from build123d import *

# Parameters (mm, degrees)
SKETCH1_W           = 498.348
SKETCH1_H           = 165.1
BOSS_EXTRUDE1_DEPTH = 1.5875
BOSS_EXTRUDE2_DEPTH = 3.175
CUT_EXTRUDE1_DEPTH  = 286.681383539
LPATTERN1_COUNT     = 5
LPATTERN1_PITCH     = 88.9
CUT_EXTRUDE2_DEPTH  = 286.681383539
LPATTERN2_COUNT     = 2
LPATTERN2_PITCH     = 38.1


with BuildPart() as part:
    # Sketch1 → Boss-Extrude1 (new, symmetric)
    with BuildSketch(Plane(origin=(0, 0, 0), x_dir=(0, 0, -1), z_dir=(1, 0, 0))):
        Rectangle(SKETCH1_W, SKETCH1_H)
    extrude(amount=BOSS_EXTRUDE1_DEPTH, both=True)

    # Sketch2 → Boss-Extrude2 (add)
    with BuildSketch(Plane(origin=(1.5875, 0, 0), x_dir=(0, 0, -1), z_dir=(1, 0, 0))):
        Polygon((192.024, -139.7), (249.174, -82.55), (-249.174, -82.55), (-249.174, -139.7), align=None)
    extrude(amount=-BOSS_EXTRUDE2_DEPTH)

    # Sketch3 → Cut-Extrude1 (cut, through all)
    with BuildSketch(Plane.ZY.offset(1.5875)):
        with BuildLine():
            ThreePointArc((222.877, -130.81), (216.603382579, -128.211382579), (219.202, -134.485))
            Line((219.202, -134.485), (219.202, -130.81))
            Line((219.202, -130.81), (222.877, -130.81))
        make_face()
        with BuildLine():
            Line((219.202, -130.81), (219.202, -134.485))
            ThreePointArc((219.202, -134.485), (221.800617421, -133.408617421), (222.877, -130.81))
            Line((222.877, -130.81), (219.202, -130.81))
        make_face()
    cut_extrude1 = extrude(amount=-CUT_EXTRUDE1_DEPTH, mode=Mode.SUBTRACT)

    # LPattern1: Cut-Extrude1 ×5
    with Locations(*[(0, 0, -i * LPATTERN1_PITCH) for i in range(1, LPATTERN1_COUNT)]):
        add(cut_extrude1, mode=Mode.SUBTRACT)

    # Sketch4 → Cut-Extrude2 (cut, symmetric)
    with BuildSketch(Plane.ZY.offset(1.5875)):
        with BuildLine():
            ThreePointArc((-194.635179285, -117.249359697), (-199.716540899, -113.854102415), (-200.908796706, -119.847977118))
            Line((-200.908796706, -119.847977118), (-198.310179285, -117.249359697))
            Line((-198.310179285, -117.249359697), (-195.711561864, -119.847977118))
            ThreePointArc((-195.711561864, -119.847977118), (-194.914922003, -118.655721311), (-194.635179285, -117.249359697))
        make_face()
        with BuildLine():
            Line((-198.310179285, -117.249359697), (-200.908796706, -119.847977118))
            ThreePointArc((-200.908796706, -119.847977118), (-198.310179285, -120.924359697), (-195.711561864, -119.847977118))
            Line((-195.711561864, -119.847977118), (-198.310179285, -117.249359697))
        make_face()
    cut_extrude2 = extrude(amount=CUT_EXTRUDE2_DEPTH, both=True, mode=Mode.SUBTRACT)

    # LPattern2: Cut-Extrude2 ×2
    with Locations(*[Vector(0, 0.7071067811865446, -0.7071067811865507) * (i * LPATTERN2_PITCH) for i in range(1, LPATTERN2_COUNT)]):
        add(cut_extrude2, mode=Mode.SUBTRACT)


solid = part.part
The model under review builds one solid part; all positions refer to its coordinate system, in mm. Give positions to 0.01 mm unless a question says otherwise; leave off trailing zeros. Order: outer loops, then holes, each group sorted by start corner. A loop starts at its lowest first (then second) coordinate and runs counter-clockwise, first axis right, second up. Notation, with made-up numbers: M 16.5,-18.5 L 70.5,-18.5 A16 cw 70.5,-14.5 Z; hole C -1.5,6 d6. An arc over 180 degrees is marked long. Answer in a Markdown table with one row per item. Add a question column.
1. For pin 1 Ø9.5 at (y, z) = (-90.31, -225.25) entering from +X; pin 2 Ø4.5 at (y, z) = (-117.25, -198.31) entering from -X, all flat-tipped, find the tip position at first contact; note any pin that passes through.
2. Add section B-B on z = -215.5. State the section outline as (x, y) points.
3. To check wall thickness, follow line 1 along Z through (x, y) = (0.3, -130.81); line 2 along Z through (x, y) = (0.5, -119); line 3 along Y through (x, z) = (-0.2, -227.5). State the ranges of each line that lie inside material, in increasing order.
4. Add section A-A on x = -0.75. State the section outline as (y, z) points (3 decimals).
The answers:
| question | item | result |
|---|---|---|
| 1 | pin 1 | x = 1.59 |
| 1 | pin 2 | through |
| 2 | outline | M -1.59,-116.22 L 1.59,-116.22 L 1.59,82.55 L -1.59,82.55 Z |
| 3 | line 1 | -200.91 to -140.07, -132.72 to -51.17, -43.82 to 37.73, 45.08 to 126.63, 133.98 to 215.53, 222.88 to 249.17 |
| 3 | line 2 | -212.72 to -201.54, -195.08 to 249.17 |
| 3 | line 3 | -104.22 to -93.22, -87.4 to 82.55 |
| 4 | outline | M -139.7,-192.024 L -82.55,-249.174 L 82.55,-249.174 L 82.55,249.174 L -139.7,249.174 Z; hole C -130.81,-136.398 d7.35; hole C -130.81,-47.498 d7.35; hole C -130.81,41.402 d7.35; hole C -130.81,130.302 d7.35; hole C -130.81,219.202 d7.35; hole C -117.249,-198.31 d7.35; hole C -90.309,-225.251 d7.35 |
